Can you work these out from the drawing? Everything is in mm from the part's minimum corner. A direction names the side the tool comes from. Coordinates: 2 decimals unless noted, no trailing zeros. Loops run counter-clockwise (first coordinate to the right, second up) from the corner with the lowest first, then second, coordinate; pieces in that order, holes last. Notation, with made-up numbers: (74.25, 23) -> (93.25, 23) arc R22 cw to (93.25, 59) -> close; hole circle Ø1 at (-22, 3). An arc over 180 degrees is marked (long way). One line per question, with ' | ' between items.
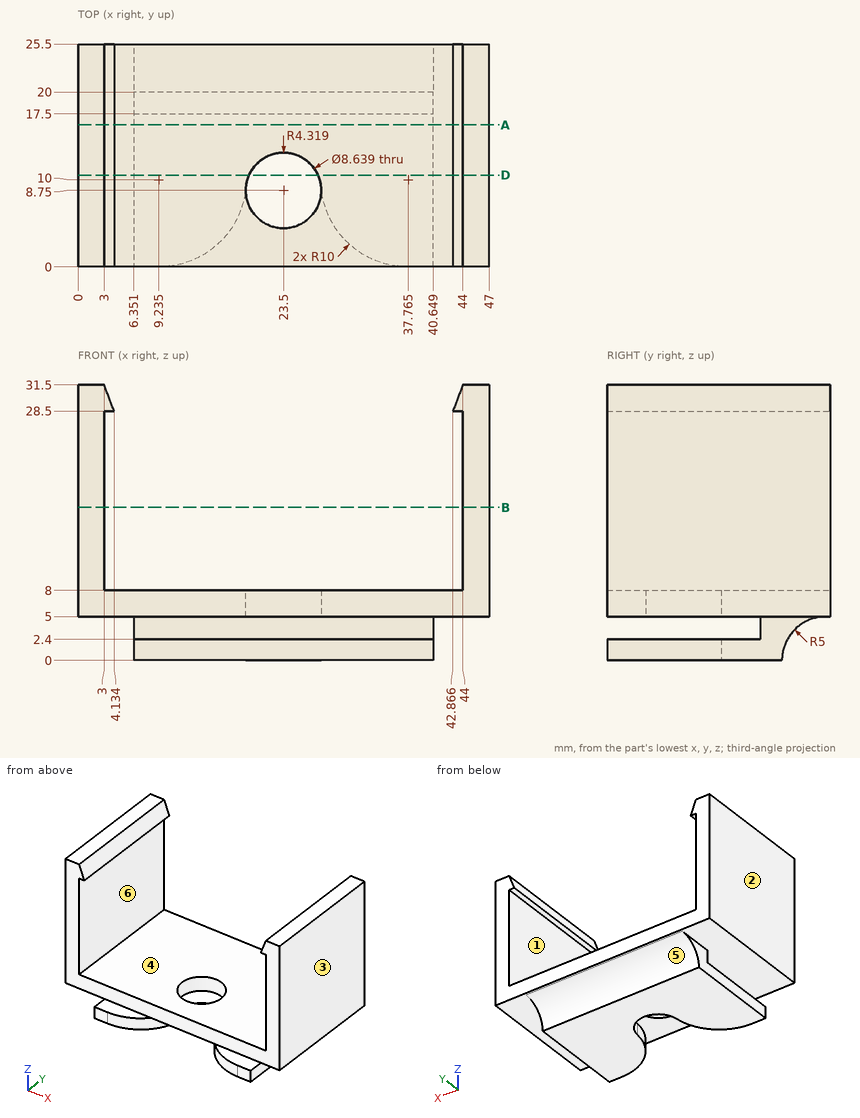
Q1. Imagine slicing it at D-D on y = 10.5. Write out the boundary of the cut face in (x, z), plus the area to 3 significant figures.
Values follow:
outline: (0, 5) -> (19.55, 5) -> (19.55, 8) -> (3, 8) -> (3, 28.5) -> (4.13, 28.5) -> (3, 31.5) -> (0, 31.5) -> close; (6.35, 0) -> (19.55, 0) -> (19.55, 2.4) -> (6.35, 2.4) -> close; (27.45, 0) -> (40.65, 0) -> (40.65, 2.4) -> (27.45, 2.4) -> close; (27.45, 5) -> (47, 5) -> (47, 31.5) -> (44, 31.5) -> (42.87, 28.5) -> (44, 28.5) -> (44, 8) -> (27.45, 8) -> close | area: 325 mm2
Q2. We'd pull the mould along X, two halves only. Please class the marked faces 3, 4, 5 and 6: released by +X, released by -X, zero draft, split by the parting line, or undercut.
Values follow:
face 3: released by +X | face 4: undercut | face 5: zero draft | face 6: undercut
Q3. Imagine slicing it at B-B on z = 17.5. Write out the boundary of the cut face in (x, y), plus the area to 3 significant figures.
Values follow:
outline: (0, 0) -> (3, 0) -> (3, 25.5) -> (0, 25.5) -> close; (44, 0) -> (47, 0) -> (47, 25.5) -> (44, 25.5) -> close | area: 153 mm2
Q4. Imagine slicing it at A-A on y = 16.25. Write out the boundary of the cut face in (x, z).
Values follow:
outline: (0, 5) -> (47, 5) -> (47, 31.5) -> (44, 31.5) -> (42.87, 28.5) -> (44, 28.5) -> (44, 8) -> (3, 8) -> (3, 28.5) -> (4.13, 28.5) -> (3, 31.5) -> (0, 31.5) -> close; (6.35, 0) -> (40.65, 0) -> (40.65, 2.4) -> (6.35, 2.4) -> close
Q5. Please list where these lines run through material, in increasing order: L1, parallel to Z at x = 33, y = 11.25; L2, parallel to Y at x = 23.5, z = 5.95; L3, parallel to Z at x = 26, y = 18. Write a range as [from, to].
Values follow:
L1: z = [0, 2.4], [5, 8] | L2: y = [0, 4.43], [13.07, 25.5] | L3: z = [0, 8]
Q6. For the marked faces 1 and 2, which set-ups out of +Z, -Z, +X, -X, +Y, -Y let a thin tool reach every point of the face, with its end or its side?
Values follow:
face 1: +Y, -Y | face 2: +Z, -Z, -X, +Y, -Y
Q7. For pin 1 (6 mm diameter, centred on x = 11, y = 11.5, fed in from +Z); pin 2 (0.9 mm diameter, centred on x = 3.5, y = 16.5, fed in from -Z); pin 3 (2.5 mm diameter, centred on y = 17, z = 1.5, fed in from +X), each with a flat end and sliding along its axis, tell me the tip position at first contact or that it passes through.
Values follow:
pin 1: stops at z = 8 | pin 2: stops at z = 5 | pin 3: stops at x = 40.65
